```python
from build123d import *

# Parameters (mm, degrees)
F0_W      = 127
F0_H      = 50.8
F1_DEPTH  = 25.4
F3_DEPTH  = 31.75
F4_R      = 5.08
F5_R      = 5.08
F6_R      = 5.08
F7_R      = 5.08
F9_DEPTH  = 25.4
F8_W      = 57.15
F8_H      = 25.4
F10_DEPTH = 25.4
F11_W     = 57.15
F11_H     = 25.4
F12_DEPTH = 25.4
F13_DEPTH = 25.4
F14_R     = 5.08


with BuildPart() as f1:
    # F0 (on Front) → F1 (new body, symmetric)
    with BuildSketch(Plane.XZ):
        Rectangle(F0_W, F0_H)
    extrude(amount=F1_DEPTH, both=True)

    # F2 (on Front) → F3 (join, symmetric)
    with BuildSketch(Plane.XZ):
        Polygon((55.5625, 31.75), (55.5625, 0), (55.5625, -31.75), (58.7375, -31.75), (58.7375, 31.75), align=None)
        Polygon((46.0375, 31.75), (46.0375, 0), (47.625, 0), (49.2125, 0), (49.2125, 31.75), align=None)
        Polygon((36.5125, 31.75), (36.5125, 0), (38.1, 0), (39.6875, 0), (39.6875, 31.75), align=None)
        Polygon((26.9875, 31.75), (26.9875, 0), (28.575, 0), (30.1625, 0), (30.1625, 31.75), align=None)
        Polygon((17.4625, 31.75), (17.4625, 0), (19.05, 0), (20.6375, 0), (20.6375, 31.75), align=None)
        Polygon((7.9375, 31.75), (7.9375, 0), (9.525, 0), (11.1125, 0), (11.1125, 31.75), align=None)
        Polygon((1.5875, 31.75), (-1.5875, 31.75), (-1.5875, -31.75), (1.5875, -31.75), (1.5875, 0), align=None)
        Polygon((9.525, 0), (7.9375, 0), (7.9375, -31.75), (11.1125, -31.75), (11.1125, 0), align=None)
        Polygon((19.05, 0), (17.4625, 0), (17.4625, -31.75), (20.6375, -31.75), (20.6375, 0), align=None)
        Polygon((28.575, 0), (26.9875, 0), (26.9875, -31.75), (30.1625, -31.75), (30.1625, 0), align=None)
        Polygon((38.1, 0), (36.5125, 0), (36.5125, -31.75), (39.6875, -31.75), (39.6875, 0), align=None)
        Polygon((47.625, 0), (46.0375, 0), (46.0375, -31.75), (49.2125, -31.75), (49.2125, 0), align=None)
    extrude(amount=F3_DEPTH, both=True)

    # F4
    f4_edges = [f1.edges().sort_by_distance(p)[0] for p in [
        (0, -31.75, 31.75),
        (9.525, -31.75, 31.75),
        (19.05, -31.75, 31.75),
        (28.575, -31.75, 31.75),
        (38.1, -31.75, 31.75),
        (47.625, -31.75, 31.75),
        (57.15, -31.75, 31.75),
    ]]
    fillet(f4_edges, radius=F4_R)

    # F5
    f5_edges = [f1.edges().sort_by_distance(p)[0] for p in [
        (0, 31.75, 31.75),
        (9.525, 31.75, 31.75),
        (19.05, 31.75, 31.75),
        (28.575, 31.75, 31.75),
        (38.1, 31.75, 31.75),
        (47.625, 31.75, 31.75),
        (57.15, 31.75, 31.75),
    ]]
    fillet(f5_edges, radius=F5_R)

    # F6
    f6_edges = [f1.edges().sort_by_distance(p)[0] for p in [
        (57.15, 31.75, -31.75),
        (47.625, 31.75, -31.75),
        (38.1, 31.75, -31.75),
        (19.05, 31.75, -31.75),
        (28.575, 31.75, -31.75),
        (9.525, 31.75, -31.75),
        (0, 31.75, -31.75),
    ]]
    fillet(f6_edges, radius=F6_R)

    # F7
    f7_edges = [f1.edges().sort_by_distance(p)[0] for p in [
        (9.525, -31.75, -31.75),
        (19.05, -31.75, -31.75),
        (28.575, -31.75, -31.75),
        (38.1, -31.75, -31.75),
        (47.625, -31.75, -31.75),
        (57.15, -31.75, -31.75),
    ]]
    fillet(f7_edges, radius=F7_R)

    # F9 (cut): a face of the model
    f9_faces = [f1.faces().sort_by_distance(p)[0] for p in [
        (-32.54375, 0, 25.4),
    ]]
    extrude(f9_faces, amount=-F9_DEPTH, mode=Mode.SUBTRACT)

    # F8 (on Top) → F10 (cut)
    with BuildSketch(Plane.XY):
        with Locations((-34.925, 12.7)):
            Rectangle(F8_W, F8_H)
    extrude(amount=-F10_DEPTH, mode=Mode.SUBTRACT)

    # F11 (on Top) → F12 (cut)
    with BuildSketch(Plane.XY):
        with Locations((-34.925, -12.7)):
            Rectangle(F11_W, F11_H)
    extrude(amount=-F12_DEPTH, mode=Mode.SUBTRACT)

    # F13 (add): a face of the model
    f13_faces = [f1.faces().sort_by_distance(p)[0] for p in [
        (-3.96875, 0, 0),
    ]]
    extrude(f13_faces, amount=F13_DEPTH)

    # F14
    f14_edges = [f1.edges().sort_by_distance(p)[0] for p in [
        (0, -31.75, -31.75),
    ]]
    fillet(f14_edges, radius=F14_R)


solid = f1.part
```
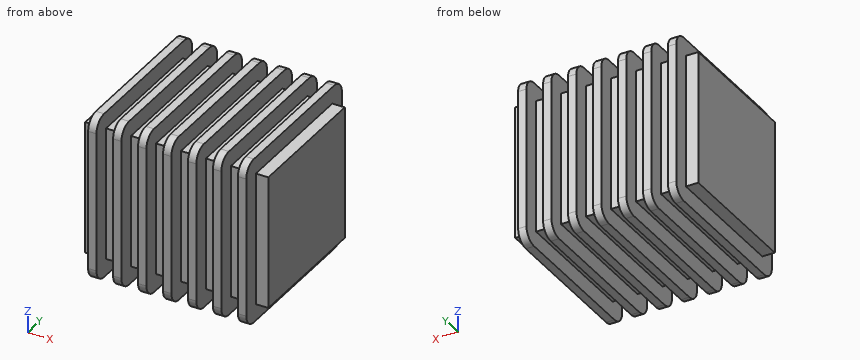
Design review of the part built by this model. Coordinates are the model's own, in mm. Coordinates: 2 decimals unless noted, no trailing zeros. Write each loop counter-clockwise with the first axis right and the second up, starting at its lowest first coordinate (ties: lowest second). Pieces come first, ordered by that corner, then holes.
1) Add section A-A (x = 31.5). Write out the cut boundary in (y, z), plus the area to 3 significant figures.
2) To check wall thickness, follow L1, parallel to Z at x = -2.5, y = -13; L2, parallel to Z at x = 0, y = 28. State the ranges of each line that lie inside material, in increasing order.
3) Insertion check: pin 1 (1.9 mm diameter, centred on x = 13.5, z = -1, fed in from +Y); pin 2 (7 mm diameter, centred on x = 43, y = -6.5, fed in from +Z); pin 3 (5 mm diameter, centred on x = 61.5, y = -3.5, fed in from +Z); pin 4 (1 mm diameter, centred on x = 44.5, z = -25.5, fed in from -Y). Each pin has a flat end and moves straight along its axis. Give the tip position at first contact, or say it passes through.
Check result:
1. outline: (-25.4, -25.4) - (25.4, -25.4) - (25.4, 25.4) - (-25.4, 25.4) - close
1. area: 2,580 mm2
2. L1: z = -25.4 to 25.4
2. L2: z = -31.57 to 31.57
3. pin 1: stops at y = 25.4
3. pin 2: stops at z = 31.75
3. pin 3: stops at z = 25.4
3. pin 4: stops at y = -25.4
